For this review, take the finished solid that the model builds, in its own axes (mm). Face numbers are marked on the shaded views. A direction names the side the tool comes from. Give positions to 0.01 mm unless a question says otherwise; leave off trailing zeros. Order: outer loops, then holes, each group sorted by start corner. A loop starts at its lowest first (then second) coordinate and runs counter-clockwise, first axis right, second up. Notation, with made-up numbers: (8.5, 78.5) - (12.5, 78.5) arc R26 ccw to (12.5, 96.5) - close; hole circle Ø7 at (-40, 16). An arc over 180 degrees is marked (long way). Answer as a JSON object with one key per item and string values. Group by question number.
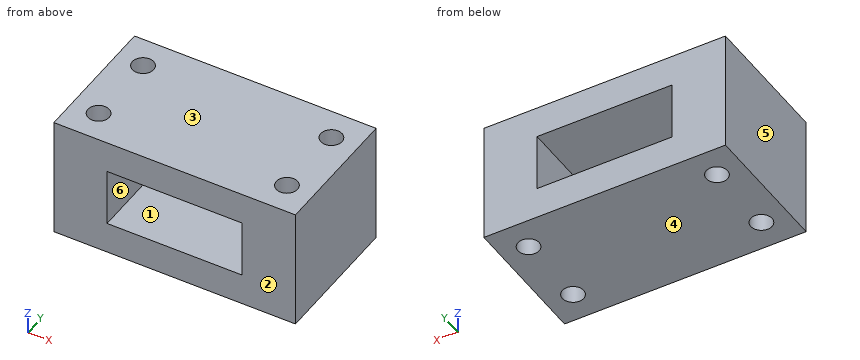
from build123d import *

# Parameters (mm, degrees)
SKETCH1_W           = 45.4
SKETCH1_H           = 22.922
SKETCH1_W_2         = 25.4
SKETCH1_H_2         = 10.922
BOSS_EXTRUDE1_DEPTH = 25.4
SKETCH2_R           = 2
CUT_EXTRUDE1_DEPTH  = 23.922


with BuildPart() as part:
    # Sketch1 → Boss-Extrude1 (new body)
    with BuildSketch(Plane(origin=(0, 0, 0), x_dir=(1, 0, 0), z_dir=(0, 1, 0))):
        Rectangle(SKETCH1_W, SKETCH1_H)
        Rectangle(SKETCH1_W_2, SKETCH1_H_2, mode=Mode.SUBTRACT)
    extrude(amount=BOSS_EXTRUDE1_DEPTH)

    # Sketch2 → Cut-Extrude1 (cut, through all)
    with BuildSketch(Plane(origin=(0, 0, -11.461), x_dir=(-1, 0, 0), z_dir=(0, 0, -1))):
        with Locations((-17.7, 5.7)):
            Circle(SKETCH2_R)
        with Locations((-17.7, 19.7)):
            Circle(SKETCH2_R)
        with Locations((17.7, 19.7)):
            Circle(SKETCH2_R)
        with Locations((17.7, 5.7)):
            Circle(SKETCH2_R)
    extrude(amount=-CUT_EXTRUDE1_DEPTH, mode=Mode.SUBTRACT)


solid = part.part
1) Consider section D-D (x = 11). Give the boundary of the cut face in (y, z), plus the area to 3 significant figures.
2) Mouldability with a two-part tool opening along Z and no side actions: class the marked faces 3, 4, 5 and 6 as released by +Z, released by -Z, zero draft, split by the parting line, or undercut.
3) For line 1 (X direction, y = 19.75, z = 9.75); line 2 (Y direction, x = 17.7, z = 7); line 3 (Z direction, x = -6, y = 16), list the stretches that pass through material, from the lowest coordinate up.
4) Consider section B-B (z = 4). Give the boundary of the cut face in (x, y).
5) Consider section A-A (y = 19.7). Give the boundary of the cut face in (x, z).
6) For the marked faces 1 and 2, list the 3-axis set-ups (+Z, -Z, +X, -X, +Y, -Y) from which the entire face can be reached by the end or side of a thin tool; tool diameter is ignored.
7) Consider section C-C (x = 17.7). Give the boundary of the cut face in (y, z).
Result set:
{
 "1": {"outline": "(0, -11.46) - (25.4, -11.46) - (25.4, -5.46) - (0, -5.46) - close; (0, 5.46) - (25.4, 5.46) - (25.4, 11.46) - (0, 11.46) - close", "area": "305 mm2"},
 "2": {"face 3": "released by +Z", "face 4": "released by -Z", "face 5": "zero draft", "face 6": "undercut"},
 "3": {"line 1": "x = -22.7 to -19.7, -15.7 to 15.7, 19.7 to 22.7", "line 2": "y = 0 to 3.7, 7.7 to 17.7, 21.7 to 25.4", "line 3": "z = -11.46 to -5.46, 5.46 to 11.46"},
 "4": {"outline": "(-22.7, 0) - (-12.7, 0) - (-12.7, 25.4) - (-22.7, 25.4) - close; (12.7, 0) - (22.7, 0) - (22.7, 25.4) - (12.7, 25.4) - close; hole circle Ø4 at (-17.7, 5.7); hole circle Ø4 at (-17.7, 19.7); hole circle Ø4 at (17.7, 5.7); hole circle Ø4 at (17.7, 19.7)"},
 "5": {"outline": "(-22.7, -11.46) - (-19.7, -11.46) - (-19.7, 11.46) - (-22.7, 11.46) - close; (-15.7, -11.46) - (15.7, -11.46) - (15.7, 11.46) - (-15.7, 11.46) - close; (19.7, -11.46) - (22.7, -11.46) - (22.7, 11.46) - (19.7, 11.46) - close; hole (-12.7, -5.46) - (12.7, -5.46) - (12.7, 5.46) - (-12.7, 5.46) - close"},
 "6": {"face 1": "+Y, -Y", "face 2": "+Z, -Z, +X, -X, -Y"},
 "7": {"outline": "(0, -11.46) - (3.7, -11.46) - (3.7, 11.46) - (0, 11.46) - close; (7.7, -11.46) - (17.7, -11.46) - (17.7, 11.46) - (7.7, 11.46) - close; (21.7, -11.46) - (25.4, -11.46) - (25.4, 11.46) - (21.7, 11.46) - close"}
}
